Check sheet for the drawn part. Datum: minimum x, y, z corner. Units: mm. A direction names the side the tool comes from. Give positions to 0.01 mm unless a question says otherwise; leave off trailing zeros. Write each loop counter-clockwise with the first axis right and the second up, starting at its lowest first coordinate (ties: lowest second). Pieces come first, ordered by that corner, then holes. Notation, with made-up numbers: (-19, 76.5) -> (-1, 76.5) arc R24 ccw to (-1, 103.5) -> close; hole circle Ø2 at (70.5, 88.5). An arc over 180 degrees is marked (long way). Write item = value, one per line. Start each with the question number.
1. Cross-section at C-C, the plane z = 6.5. Record the cut outline in (x, y), plus the area to 3 significant figures.
2. Depth check by flat-ended pin: P1, Ø3, axis at x = 16.5, z = 8, coming from the +Y side; P2, Ø5, axis at x = 12.1, y = 12.1, coming from the +Z side; P3, Ø6, axis at y = 7, z = 6, coming from the -X side; P4, Ø10, axis at x = 17.5, y = 13, coming from the +Z side. Enter the tip coordinate at first touch or a pass-through.
3. Thickness scan on line 1 along Y through (x, z) = (12.1, 5.75); line 2 along Z through (x, y) = (10.25, 19.75); line 3 along Z through (x, y) = (3, 9). Record the ranges inside material, lowest first.
4. Cross-section at A-A, the plane x = 12.1. Record the cut outline in (y, z).
5. Mould release check, pull along Y, two halves, no side actions. Record for the marked faces 1, 2 and 3: pulls with the +Y half, pulls with the -Y half, needs draft (parallel to the pull), parting line crosses it, or undercut.
6. Set-up check for the marked faces 4 and 5: record each of +Z, -Z, +X, -X, +Y, -Y from which the full face is reachable in a straight line by a thin tool's end or side.
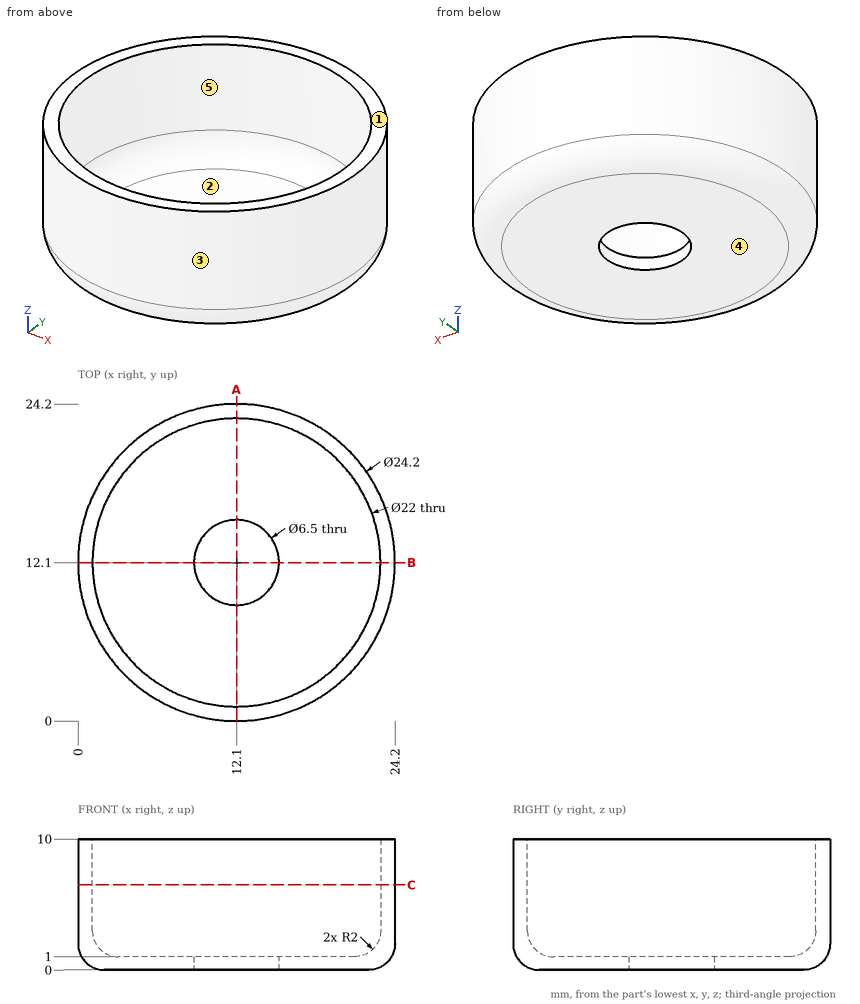
Answers:
q1.outline = circle Ø24.2 at (12.1, 12.1); hole circle Ø22 at (12.1, 12.1)
q1.area = 79.8 mm^2
q2.P1 = 23.85
q2.P2 = through
q2.P3 = 0.18
q2.P4 = 1.65
q3.line_1 = 0 to 1.1, 23.1 to 24.2
q3.line_2 = 0 to 1
q3.line_3 = 0 to 1.1
q4.outline = (0, 2) arc R2 ccw to (2, 0) -> (8.85, 0) -> (8.85, 1) -> (3.1, 1) arc R2 cw to (1.1, 3) -> (1.1, 10) -> (0, 10) -> close; (15.35, 0) -> (22.2, 0) arc R2 ccw to (24.2, 2) -> (24.2, 10) -> (23.1, 10) -> (23.1, 3) arc R2 cw to (21.1, 1) -> (15.35, 1) -> close
q5.face_1 = needs draft
q5.face_2 = undercut
q5.face_3 = parting line crosses it
q6.face_4 = -Z, +X, -X, +Y, -Y
q6.face_5 = +Z
